```python
from build123d import *

# Parameters (mm, degrees)
F0_W     = 50
F0_H     = 50
F0_R     = 2
F0_W_2   = 35
F0_H_2   = 35
F1_DEPTH = 2.5
F2_R     = 3
F3_SIZE  = 0.5
F4_R     = 0.99999


# Not quite as in the source:
# - a fillet or chamfer is up to 0.001 mm smaller than in the source, because OpenCascade refuses the exact size


with BuildPart() as f1:
    # F0 (on Top) → F1 (new body)
    with BuildSketch(Plane.XY):
        with Locations((11.1718769372, 3.8648895919)):
            Rectangle(F0_W, F0_H)
        with Locations((-10.3281230628, -17.6351104081)):
            Circle(F0_R, mode=Mode.SUBTRACT)
        with Locations((32.6718769372, -17.6351104081)):
            Circle(F0_R, mode=Mode.SUBTRACT)
        with Locations((11.1718769372, 3.8648895919)):
            Rectangle(F0_W_2, F0_H_2, mode=Mode.SUBTRACT)
        with Locations((-10.3281230628, 25.3648895919)):
            Circle(F0_R, mode=Mode.SUBTRACT)
        with Locations((32.6718769372, 25.3648895919)):
            Circle(F0_R, mode=Mode.SUBTRACT)
    extrude(amount=F1_DEPTH)

    # F2
    f2_edges = [f1.edges().sort_by_distance(p)[0] for p in [
        (-13.828123, 28.86489, 1.25),
        (36.171877, 28.86489, 1.25),
        (36.171877, -21.13511, 1.25),
        (-13.828123, -21.13511, 1.25),
    ]]
    fillet(f2_edges, radius=F2_R)

    # F3
    f3_edges = [f1.edges().sort_by_distance(p)[0] for p in [
        (-12.328123, 25.36489, 2.5),
        (30.671877, 25.36489, 2.5),
        (30.671877, -17.63511, 2.5),
        (-12.328123, -17.63511, 2.5),
    ]]
    chamfer(f3_edges, length=F3_SIZE)

    # F4 (radius 1 in the source; OpenCascade refuses exactly that, so slightly less here)
    f4_edges = [f1.edges().sort_by_distance(p)[0] for p in [
        (11.171877, 28.86489, 2.5),
    ]]
    fillet(f4_edges, radius=F4_R)


solid = f1.part
```
Geometry: final body of the model. Coordinates: model frame, mm. A direction names the side the tool comes from. Give positions to 0.01 mm unless a question says otherwise; leave off trailing zeros. Order: outer loops, then holes, each group sorted by start corner. A loop starts at its lowest first (then second) coordinate and runs counter-clockwise, first axis right, second up. Notation, with made-up numbers: M 0,-30 L 57,-30 A25 ccw 57,5 Z; hole C 59.25,35.5 d10. An arc over 180 degrees is marked long. Answer as CSV lines item,"result". Start each with the question number.
1) Set-up query: faces 1 (the flat face through (30, 2, 0)), 2 (the flat face through (11, -13.635, 1)). Return all of +Z, -Z, +X, -X, +Y, -Y with unobstructed straight access to the full face (end or side cutting, diameter ignored); none if empty.
2) Cut plane A-A (x = -4). Output: boundary loops of the cut face in (y, z).
3) Mould query, pull axis X, two halves, no side actions, for faces 3 (the flat face through (-6.328, 4, 1)), 4 (the cylindrical face through (-12.973, -20.233, 0.761)), 5 (the flat face through (36.172, 4, 1)). Classes: +X half, -X half, draft (parallel to the pull), parting line (faces both ways), or undercut.
4) Cut plane B-B (y = 16.5). Output: boundary loops of the cut face in (x, z), then the cut area to 3 significant figures.
5) Line query: line 1 (Y direction, x = 12, z = 0.65); line 2 (X direction, y = 9, z = 1.5); line 3 (Y direction, x = 34.5, z = 1.85). Output: solid intervals per line, ascending. Write a range as from..to.
6) Cut plane C-C (z = 0.85). Output: boundary loops of the cut face in (x, y).
7) First-contact query: P1, Ø0.8, axis at y = -2.5, z = 2, coming from the -X side. Flat tip, straight axial feed; report the tip coordinate or a pass-through.
Findings below:
1,face 1,"-Z, +X, -X, +Y, -Y"
1,face 2,"+Z, -Z"
2,outline,"M -21.14,0 L -13.64,0 L -13.64,2.5 L -20.14,2.5 A1 ccw -21.14,1.5 Z; M 21.36,0 L 28.86,0 L 28.86,1.5 A1 ccw 27.86,2.5 L 21.36,2.5 Z"
3,face 3,"undercut"
3,face 4,"-X half"
3,face 5,"+X half"
4,outline,"M -13.83,0 L -6.33,0 L -6.33,2.5 L -12.83,2.5 A1 ccw -13.83,1.5 Z; M 28.67,0 L 36.17,0 L 36.17,1.5 A1 ccw 35.17,2.5 L 28.67,2.5 Z"
4,area,"37.1 mm²"
5,line 1,"y = -21.14..-13.64, 21.36..28.86"
5,line 2,"x = -13.83..-6.33, 28.67..36.17"
5,line 3,"y = -20.75..-18.45, -16.82..24.55, 26.18..28.48"
6,outline,"M -13.83,-18.14 A3 ccw -10.83,-21.14 L 33.17,-21.14 A3 ccw 36.17,-18.14 L 36.17,25.86 A3 ccw 33.17,28.86 L -10.83,28.86 A3 ccw -13.83,25.86 Z; hole C -10.33,-17.64 d4; hole C -10.33,25.36 d4; hole M -6.33,-13.64 L 28.67,-13.64 L 28.67,21.36 L -6.33,21.36 Z; hole C 32.67,-17.64 d4; hole C 32.67,25.36 d4"
7,P1,"stops at x = -13.82"
